```python
from build123d import *

# Parameters (mm, degrees)
EXTRUDE_1_DEPTH          = 2.7
EXTRUDE_1_DEPTH_BACK     = 2.7
EXTRUDE_2_DEPTH          = 1
EXTRUDE_2_DEPTH_BACK     = 1
CUT_EXTRUDE_1_DEPTH      = 22.678099548
PATTERN_LINEAR_1_COUNT   = 2
PATTERN_LINEAR_1_PITCH   = 7.5
EXTRUDE_3_DEPTH          = 2
EXTRUDE_3_DEPTH_BACK     = 2
CUT_EXTRUDE_2_DEPTH      = 2
CUT_EXTRUDE_2_DEPTH_BACK = 2
FILLET_1_R               = 0.1
FILLET_4_R               = 0.2
FILLET_5_R               = 0.2
FILLET_7_R               = 0.2


with BuildPart() as part:
    # 草图1 → 凸台-拉伸1 (new, two sides: drawn at the far end of the back side and taken through both)
    with BuildSketch(Plane.XY.offset(-EXTRUDE_1_DEPTH_BACK)):
        Polygon((0, 0), (7.5, 0), (7.5, 2), (-7.5, 2), (-7.5, 0), align=None)
    extrude(amount=EXTRUDE_1_DEPTH + EXTRUDE_1_DEPTH_BACK)

    # 草图2 → 凸台-拉伸2 (add, two sides: drawn at the far end of the back side and taken through both)
    with BuildSketch(Plane.XY.offset(-EXTRUDE_2_DEPTH_BACK)):
        with BuildLine():
            Line((-7.5, 2), (-4.91592968, 15.913036354))
            ThreePointArc((-4.91592968, 15.913036354), (0, 20), (4.91592968, 15.913036354))
            Line((4.91592968, 15.913036354), (7.5, 2))
            Line((7.5, 2), (-7.5, 2))
        make_face()
    extrude(amount=EXTRUDE_2_DEPTH + EXTRUDE_2_DEPTH_BACK)

    # 草图3 → 切除-拉伸1 (cut, through all)
    with BuildSketch(Plane.XY.offset(1)):
        with BuildLine():
            Line((3.5, 6), (3.5, 9))
            Line((3.5, 9), (1.322875656, 9))
            ThreePointArc((1.322875656, 9), (0, 9.5), (-1.322875656, 9))
            Line((-1.322875656, 9), (-3.5, 9))
            Line((-3.5, 9), (-3.5, 6))
            Line((-3.5, 6), (-1.322875656, 6))
            ThreePointArc((-1.322875656, 6), (0, 5.5), (1.322875656, 6))
            Line((1.322875656, 6), (3.5, 6))
        make_face()
    cut_extrude_1 = extrude(amount=-CUT_EXTRUDE_1_DEPTH, mode=Mode.SUBTRACT)

    # 阵列(线性)1: 切除-拉伸1 ×2
    with Locations(*[(0, i * PATTERN_LINEAR_1_PITCH, 0) for i in range(1, PATTERN_LINEAR_1_COUNT)]):
        add(cut_extrude_1, mode=Mode.SUBTRACT)

    # 草图4 → 凸台-拉伸3 (add, two sides: drawn at the far end of the back side and taken through both)
    with BuildSketch(Plane.XY.offset(-EXTRUDE_3_DEPTH_BACK)):
        with BuildLine():
            Line((1.5, 0), (-1.5, 0))
            Line((-1.5, 0), (-1.5, -0.677124344))
            ThreePointArc((-1.5, -0.677124344), (-1.780042303, -1.088161527), (-1.95, -1.555590279))
            Line((-1.95, -1.555590279), (-1.95, -2.5))
            Line((-1.95, -2.5), (1.95, -2.5))
            Line((1.95, -2.5), (1.95, -1.555590279))
            ThreePointArc((1.95, -1.555590279), (1.780042303, -1.088161527), (1.5, -0.677124344))
            Line((1.5, -0.677124344), (1.5, 0))
        make_face()
    extrude(amount=EXTRUDE_3_DEPTH + EXTRUDE_3_DEPTH_BACK)

    # 草图5 → 切除-拉伸2 (cut, two sides: drawn at the far end of the back side and taken through both)
    with BuildSketch(Plane(origin=(0, 0, 0), x_dir=(0, 0, -1), z_dir=(1, 0, 0)).offset(-CUT_EXTRUDE_2_DEPTH_BACK)):
        with BuildLine():
            Line((1.5, 0), (1.5, -0.677124344))
            ThreePointArc((1.5, -0.677124344), (1.780042303, -1.088161527), (1.95, -1.555590279))
            Line((1.95, -1.555590279), (1.95, -2.5))
            Line((1.95, -2.5), (2, -2.5))
            Line((2, -2.5), (2, 0))
            Line((2, 0), (1.5, 0))
        make_face()
        with BuildLine():
            Line((-2, 0), (-1.5, 0))
            Line((-1.5, 0), (-1.5, -0.677124344))
            ThreePointArc((-1.5, -0.677124344), (-1.780042303, -1.088161527), (-1.95, -1.555590279))
            Line((-1.95, -1.555590279), (-1.95, -2.5))
            Line((-1.95, -2.5), (-2, -2.5))
            Line((-2, -2.5), (-2, 0))
        make_face()
    extrude(amount=CUT_EXTRUDE_2_DEPTH + CUT_EXTRUDE_2_DEPTH_BACK, mode=Mode.SUBTRACT)

    # 圆角1
    fillet_1_edges = [part.edges().sort_by_distance(p)[0] for p in [
        (-1.95, -2.5, 0),
        (1.95, -2.5, 0),
        (0, -2.5, -1.95),
        (0, -2.5, 1.95),
    ]]
    fillet(fillet_1_edges, radius=FILLET_1_R)

    # 圆角4
    fillet_4_edges = [part.edges().sort_by_distance(p)[0] for p in [
        (-7.5, 1, 2.7),
        (0, 2, 2.7),
        (7.5, 1, 2.7),
        (0, 0, 2.7),
        (7.5, 1, -2.7),
        (0, 2, -2.7),
        (-7.5, 1, -2.7),
        (0, 0, -2.7),
    ]]
    fillet(fillet_4_edges, radius=FILLET_4_R)

    # 圆角5
    # the kernel refuses this fillet: 0.2 mm, written as the material it takes off along each edge
    with BuildSketch(Plane(origin=(7.3, 0.2, 2.5), x_dir=(1, 0, 0), z_dir=(0, -1, 0))) as fillet_5_piece_1_section:
        Polygon((0, 0), (FILLET_5_R, 0), (FILLET_5_R, FILLET_5_R), (0, FILLET_5_R), align=None)
    fillet_5_piece_1 = extrude(amount=FILLET_5_R, mode=Mode.PRIVATE)
    fillet_5_piece_1 = fillet_5_piece_1 - Plane(origin=(7.3, 0.2, 2.5), x_dir=(-0.7071067811865475, 0, -0.7071067811865475), z_dir=(0, -1, 0)) * Sphere(FILLET_5_R, mode=Mode.PRIVATE)
    add(fillet_5_piece_1, mode=Mode.SUBTRACT)
    with BuildSketch(Plane(origin=(-7.3, 0.2, 2.5), x_dir=(-1, 0, 0), z_dir=(0, -1, 0))) as fillet_5_piece_2_section:
        Polygon((0, 0), (FILLET_5_R, 0), (FILLET_5_R, -FILLET_5_R), (0, -FILLET_5_R), align=None)
    fillet_5_piece_2 = extrude(amount=FILLET_5_R, mode=Mode.PRIVATE)
    fillet_5_piece_2 = fillet_5_piece_2 - Plane(origin=(-7.3, 0.2, 2.5), x_dir=(0.7071067811865475, 1.2560739669470211e-15, -0.7071067811865475), z_dir=(0, -1, 0)) * Sphere(FILLET_5_R, mode=Mode.PRIVATE)
    add(fillet_5_piece_2, mode=Mode.SUBTRACT)
    with BuildSketch(Plane(origin=(-7.3, 0.2, -2.5), x_dir=(-1, 0, 0), z_dir=(0, -1, 0))) as fillet_5_piece_3_section:
        Polygon((0, 0), (FILLET_5_R, 0), (FILLET_5_R, FILLET_5_R), (0, FILLET_5_R), align=None)
    fillet_5_piece_3 = extrude(amount=FILLET_5_R, mode=Mode.PRIVATE)
    fillet_5_piece_3 = fillet_5_piece_3 - Plane(origin=(-7.3, 0.2, -2.5), x_dir=(0.7071067811865475, 1.2560739669470211e-15, 0.7071067811865475), z_dir=(0, -1, 0)) * Sphere(FILLET_5_R, mode=Mode.PRIVATE)
    add(fillet_5_piece_3, mode=Mode.SUBTRACT)
    with BuildSketch(Plane(origin=(7.3, 0.2, -2.5), x_dir=(1, 0, 0), z_dir=(0, -1, 0))) as fillet_5_piece_4_section:
        Polygon((0, 0), (FILLET_5_R, 0), (FILLET_5_R, -FILLET_5_R), (0, -FILLET_5_R), align=None)
    fillet_5_piece_4 = extrude(amount=FILLET_5_R, mode=Mode.PRIVATE)
    fillet_5_piece_4 = fillet_5_piece_4 - Plane(origin=(7.3, 0.2, -2.5), x_dir=(-0.7071067811865475, 0, 0.7071067811865475), z_dir=(0, -1, 0)) * Sphere(FILLET_5_R, mode=Mode.PRIVATE)
    add(fillet_5_piece_4, mode=Mode.SUBTRACT)
    with BuildSketch(Plane(origin=(-7.5, 0, 2.5), x_dir=(1, 0, 0), z_dir=(0, 0, -1)), Plane(origin=(7.5, 0, -2.5), x_dir=(-1, 0, 0), z_dir=(0, 0, 1))) as fillet_5_piece_5:
        with BuildLine():
            CenterArc((FILLET_5_R, -FILLET_5_R), FILLET_5_R, 90, 90)
            Line((0, -FILLET_5_R), (0, 0))
            Line((0, 0), (FILLET_5_R, 0))
        make_face()
    extrude(amount=5, mode=Mode.SUBTRACT)

    # 圆角7
    fillet_7_edges = [part.edges().sort_by_distance(p)[0] for p in [
        (6.20796484, 8.956518177, 1),
        (0, 20, 1),
        (-6.20796484, 8.956518177, 1),
        (-6.20796484, 8.956518177, -1),
        (0, 20, -1),
        (6.20796484, 8.956518177, -1),
    ]]
    fillet(fillet_7_edges, radius=FILLET_7_R)


solid = part.part
```
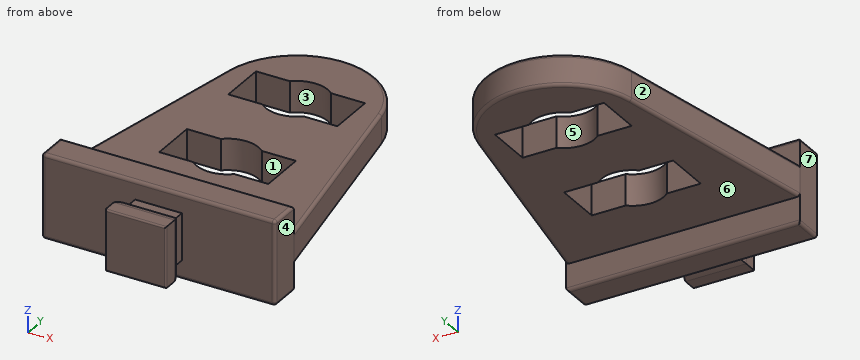
Could you check a few things on this model? Use its own coordinates, in mm. Face numbers are marked on the shaded views. A direction names the side the tool comes from. Give positions to 0.01 mm unless a question says otherwise; leave off trailing zeros. Write each loop counter-clockwise with the first axis right and the second up, starting at its lowest first coordinate (ties: lowest second). Pieces come first, ordered by that corner, then holes. Notation, with made-up numbers: (-19, 15) - (25, 15) arc R14 ccw to (25, 19) - close; hole circle Ø1 at (-23.5, -38.5). An arc over 180 degrees is marked (long way). One line per item, written item: value. Start each with the question number.
Item 1: Imagine slicing it at B-B, the plane z = 2.2. List the corners of the cut face in (x, y) for me.
Item 2: Which directions (+Z, -Z, +X, -X, +Y, -Y) give clear straight access to the entire face, cutting with the end or side of a thin tool? Please do the marked faces 5, 6 and 7.
Item 3: I'm going to push flat-ended pins straight in: pin 1 (8 mm diameter, centred on x = -4, y = 7.5, fed in from +Z); pin 2 (0.6 mm diameter, centred on x = -3, z = -0.5, fed in from -Y); pin 3 (1 mm diameter, centred on x = 2.5, z = 0, fed in from +Y). Where does each tip first touch, or does it pass through?
Item 4: Imagine slicing it at A-A, the plane z = -0.45. Give the number of separate pieces and of enclosed holes in the cut face, and give its area (3 significant figures).
Item 5: Please list where these lines run through material, in increasing order: line 1 (Y direction, x = 2.5, z = 0.55); line 2 (Z direction, x = -2, y = 5.25); line 3 (Y direction, x = -6, z = 1.2). Write a range as from..to.
Item 6: If we mould it in two halves opening along Y, with no side actions, what happens to the marked faces 1, 2, 3 and 4? For each: +Y half, -Y half, draft (parallel to the pull), parting line (faces both ways), or undercut.
Geometry says:
1. outline: (-7.5, 0.2) arc R0.2 ccw to (-7.3, 0) - (7.3, 0) arc R0.2 ccw to (7.5, 0.2) - (7.5, 2) - (-7.5, 2) - close
2. face 5: +Z, -Z
2. face 6: -Z, +X, -X, +Y
2. face 7: +Z, -Z, -X, +Y, -Y
3. pin 1: z = 1
3. pin 2: y = 0
3. pin 3: y = 19.58
4. separate pieces: 1
4. enclosed holes: 2
4. area: 196 mm^2
5. line 1: 0..6, 9..13.5, 16.5..19.33
5. line 2: -1..1
5. line 3: 0..2
6. face 1: undercut
6. face 2: +Y half
6. face 3: undercut
6. face 4: draft
